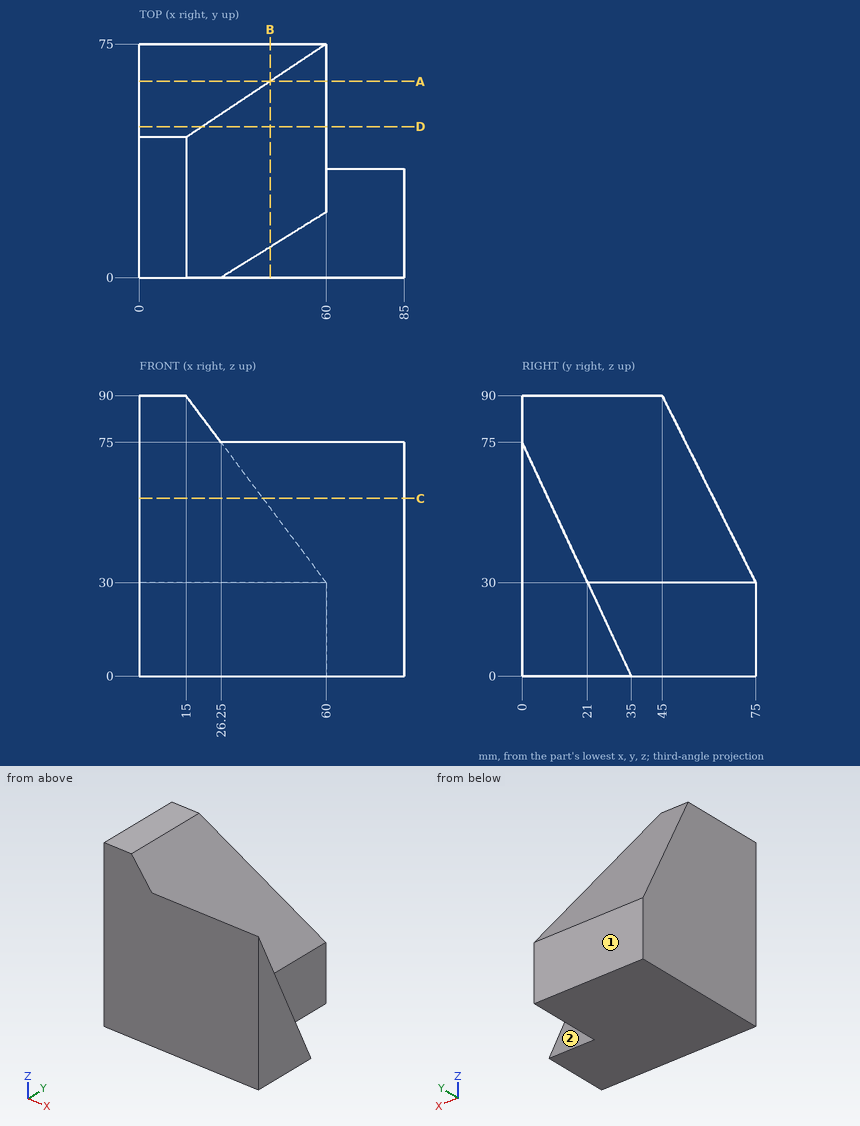
Job drawing, mm, ordinate dimensions from the low corner. One solid piece. A direction names the side the tool comes from. Coordinates: 2 decimals unless noted, no trailing zeros. Loops run counter-clockwise (first coordinate to the right, second up) from the corner with the lowest first, then second, coordinate; pieces in that order, holes last. Notation, with made-up numbers: (73, -14.5) - (83, -14.5) arc R26 ccw to (83, 23.5) - close; hole circle Ø3 at (79.5, 18). An arc over 180 degrees is marked (long way). Answer as a JSON object with one key per item and string values. Group by question number.
(1) Cut at D-D (y = 48.5). Give the cut face in (x, z), then the cut area to 3 significant figures.
(2) Tool access for the marked faces 1 and 2: list every direction of +Z, -Z, +X, -X, +Y, -Y with a clear straight run to the whole face (end or side of a thin tool).
(3) Flat gauge pins, fed straight in: pin 1 (1 mm diameter, centred on x = 72, y = 17, fed in from +Z); pin 2 (1 mm diameter, centred on x = 9.5, y = 55.5, fed in from +Z). Where does each tip first touch, or does it go through?
(4) Probe line 1 along X through (y, z) = (42, 11.5); line 2 along Z through (x, y) = (32, 38); line 3 along X through (y, z) = (20, 38.5) (3 decimals). List the from-to ranges inside material, lowest first.
(5) Cut at C-C (z = 57). Give the cut face in (x, y).
(6) Cut at B-B (x = 42). Give the cut face in (y, z), then the cut area to 3 significant figures.
(7) Cut at A-A (y = 63). Give the cut face in (x, z), then the cut area to 3 significant figures.
Geometry says:
{
 "1": {"outline": "(0, 0) - (60, 0) - (60, 30) - (20.25, 83) - (0, 83) - close", "area": "3,930 mm^2"},
 "2": {"face 1": "+Z, -Z, +X, -X, +Y", "face 2": "+Z, +X, +Y"},
 "3": {"pin 1": "stops at z = 39.64", "pin 2": "stops at z = 70"},
 "4": {"line 1": "x = 0 to 60", "line 2": "z = 0 to 67.33", "line 3": "x = 0 to 53.625"},
 "5": {"outline": "(0, 0) - (85, 0) - (85, 8.4) - (39.75, 8.4) - (39.75, 61.5) - (0, 61.5) - close"},
 "6": {"outline": "(0, 0) - (75, 0) - (75, 30) - (63, 54) - (9.8, 54) - (0, 75) - close", "area": "4,010 mm^2"},
 "7": {"outline": "(0, 0) - (60, 0) - (60, 30) - (42, 54) - (0, 54) - close", "area": "3,020 mm^2"}
}
